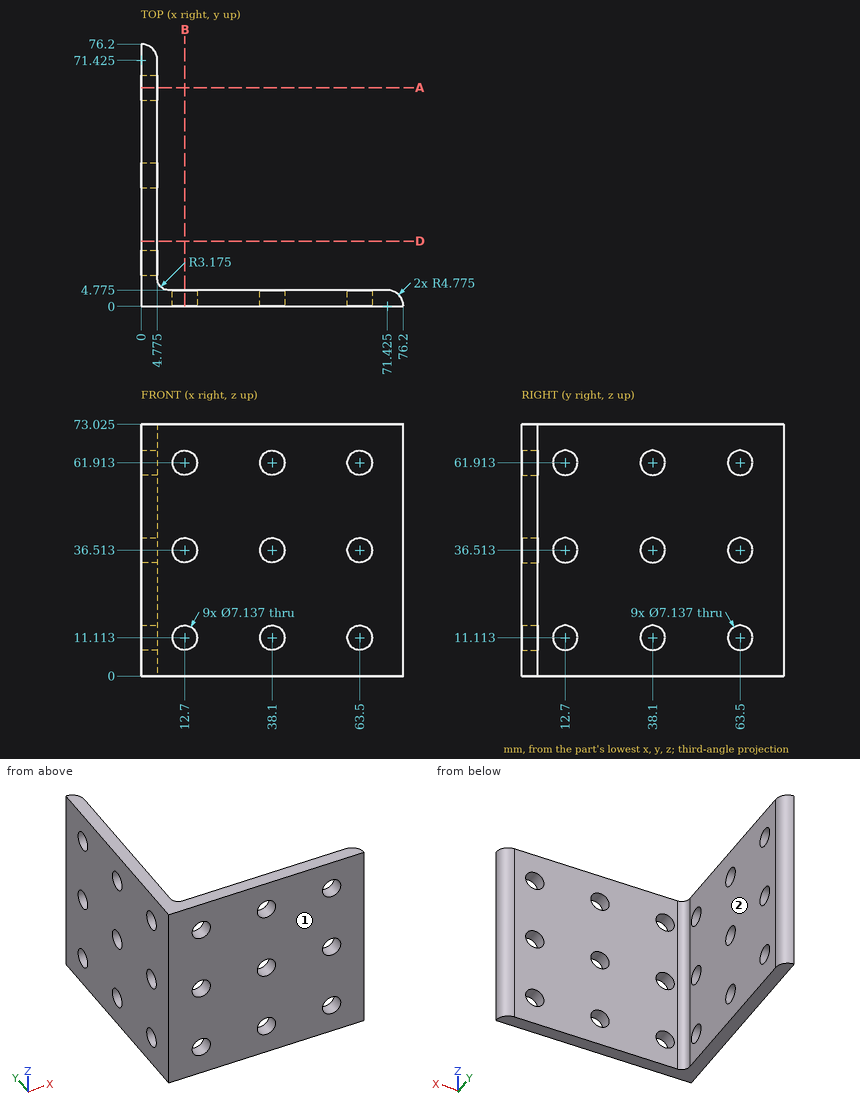
Input: dimensioned drawing with shaded views. Units: mm. Origin: part minimum x, y, z. A direction names the side the tool comes from. Coordinates: 2 decimals unless noted, no trailing zeros. Order: outer loops, then holes, each group sorted by start corner. A loop starts at its lowest first (then second) coordinate and runs counter-clockwise, first axis right, second up.
(1) Material intervals for probe 1 along Z at (x, y) = (12, 2) (1 decimal); probe 2 along X at (y, z) = (28, 30.5) (1 decimal), sorted ascending.
(2) Section query D-D (y = 19). Return the cut outline in (x, z) (1 decimal), plus the area to 3 significant figures.
(3) Section query A-A (y = 63.5). Return the cut outline in (x, z) (1 decimal).
(4) Access query for the marked faces 1 and 2. Directions: +Z, -Z, +X, -X, +Y, -Y. A direction counts if a zero-diameter tool reaches every point of the face in a straight line with its end or side. Return the directions, or none.
(5) First-contact query: pin 1 (4.5 mm diameter, centred on y = 63.5, z = 11.11, fed in from -X); pin 2 (10 mm diameter, centred on x = 34.5, z = 30, fed in from +Y) (1 decimal); pin 3 (8 mm diameter, centred on y = 12.7, z = 11.11, fed in from +X) (1 decimal); pin 4 (3 mm diameter, centred on y = 49, z = 48.5, fed in from -X). Flat tips, straight axial feed; report the tip coordinate or a pass-through.
Solution:
1. probe 1: z = 0 to 7.6, 14.6 to 33, 40 to 58.4, 65.4 to 73
1. probe 2: x = 0 to 4.8
2. outline: (0, 0) - (4.8, 0) - (4.8, 73) - (0, 73) - close
2. area: 349 mm2
3. outline: (0, 0) - (4.8, 0) - (4.8, 7.5) - (0, 7.5) - close; (0, 14.7) - (4.8, 14.7) - (4.8, 32.9) - (0, 32.9) - close; (0, 40.1) - (4.8, 40.1) - (4.8, 58.3) - (0, 58.3) - close; (0, 65.5) - (4.8, 65.5) - (4.8, 73) - (0, 73) - close
4. face 1: +Z, -Z, +X, -X, -Y
4. face 2: +Z, -Z, +X, +Y
5. pin 1: passes through
5. pin 2: stops at y = 4.8
5. pin 3: stops at x = 4.8
5. pin 4: stops at x = 0
